Design review of the part built by this model. Coordinates are the model's own, in mm. A direction names the side the tool comes from. Give positions to 0.01 mm unless a question says otherwise; leave off trailing zeros. Loops run counter-clockwise (first coordinate to the right, second up) from the corner with the lowest first, then second, coordinate; pieces in that order, holes last. Notation, with made-up numbers: (-6.75, -25) -> (9.25, -25) arc R33 ccw to (9.25, 7) -> close; hole circle Ø4 at (39, 38). An arc over 180 degrees is marked (long way). Use a Markdown table: item, result. Add a question column.
1. Add section B-B (y = 4.5). State the section outline as (x, z) points, and give its area (3 significant figures).
2. Add section A-A (x = 24). State the section outline as (y, z) points, and give its area (3 significant figures).
3. Add section D-D (x = 13). State the section outline as (y, z) points.
4. For faces 1 (the cylindrical face through (18.797, 6.859, 2.535)), 2 (the flat face through (20, 12.5, 2)), 3 (the flat face through (8, 28, 3)), list the 3-axis set-ups (+Z, -Z, +X, -X, +Y, -Y) from which the entire face can be reached by the end or side of a thin tool; tool diameter is ignored.
5. Add section C-C (z = 4.55). Count the separate pieces of the cut face and the enclosed holes in it, and give its area (3 significant figures).
6. For pin 1 Ø2 at (x, z) = (12.5, 1.5) entering from +Y; pin 2 Ø1.5 at (x, z) = (32, 3.5) entering from -Y; pin 3 Ø1.2 at (y, z) = (1.5, 3.5) entering from +X, all flat-tipped, find the tip position at first contact; note any pin that passes through.
7. Draft analysis for pull direction Y (two halves, no side actions). For faces 4 (the cylindrical face through (10.59, 16.94, 2.46)), 5 (the flat face through (18, 12, 0)), 6 (the flat face through (23.9, 0, 0.8)), state which applies: pulls with the +Y half, pulls with the -Y half, needs draft (parallel to the pull), parting line crosses it, or undercut.
8. To check wall thickness, follow line 1 (X direction, y = 10, z = 2.5); line 2 (Y direction, x = 26.5, z = 3.85); line 3 (X direction, y = 19.5, z = 1.85). State the ranges of each line that lie inside material, in increasing order.
```python
from build123d import *

# Parameters (mm, degrees)
SKETCH1_R           = 2
BOSS_EXTRUDE1_DEPTH = 5
SKETCH2_R           = 1.5
CUT_EXTRUDE1_DEPTH  = 31
CUT_EXTRUDE2_DEPTH  = 6.0000001


with BuildPart() as part:
    # Sketch1 → Boss-Extrude1 (new body)
    with BuildSketch(Plane.XY):
        with BuildLine():
            Line((1, 0), (35, 0))
            ThreePointArc((35, 0), (35.707106781, 0.292893219), (36, 1))
            Line((36, 1), (36, 29))
            ThreePointArc((36, 29), (35.707106781, 29.707106781), (35, 30))
            Line((35, 30), (1, 30))
            ThreePointArc((1, 30), (0.292893219, 29.707106781), (0, 29))
            Line((0, 29), (0, 7))
            Line((0, 7), (0, 1))
            ThreePointArc((0, 1), (0.292893219, 0.292893219), (1, 0))
        make_face()
        with Locations((5, 15)):
            Circle(SKETCH1_R, mode=Mode.SUBTRACT)
        with BuildLine():
            Line((11.967452223, 12.5), (28.032547777, 12.5))
            ThreePointArc((28.032547777, 12.5), (29.423746586, 13.076253414), (30, 14.467452223))
            Line((30, 14.467452223), (30, 15.532547777))
            ThreePointArc((30, 15.532547777), (29.423746586, 16.923746586), (28.032547777, 17.5))
            Line((28.032547777, 17.5), (11.967452223, 17.5))
            ThreePointArc((11.967452223, 17.5), (10.576253414, 16.923746586), (10, 15.532547777))
            Line((10, 15.532547777), (10, 14.467452223))
            ThreePointArc((10, 14.467452223), (10.576253414, 13.076253414), (11.967452223, 12.5))
        make_face(mode=Mode.SUBTRACT)
    extrude(amount=BOSS_EXTRUDE1_DEPTH)

    # Sketch2 → Cut-Extrude1 (cut, through all)
    with BuildSketch(Plane(origin=(0, 30, 0), x_dir=(1, 0, 0), z_dir=(0, 1, 0))):
        with Locations((4, -2.5)):
            Circle(SKETCH2_R)
        with Locations((24, -2.5)):
            Circle(SKETCH2_R)
    extrude(amount=-CUT_EXTRUDE1_DEPTH, mode=Mode.SUBTRACT)

    # Sketch3 → Cut-Extrude2 (cut, through all)
    with BuildSketch(Plane.XY.offset(5)):
        with BuildLine():
            Line((28, 30), (28, 25))
            ThreePointArc((28, 25), (28.292893219, 24.292893219), (29, 24))
            Line((29, 24), (43, 24))
            ThreePointArc((43, 24), (43.707106781, 23.707106781), (44, 23))
            Line((44, 23), (44, 7))
            ThreePointArc((44, 7), (43.707106781, 6.292893219), (43, 6))
            Line((43, 6), (29, 6))
            ThreePointArc((29, 6), (28.292893219, 5.707106781), (28, 5))
            Line((28, 5), (28, 0))
            Line((28, 0), (56.755309453, 0))
            Line((56.755309453, 0), (56.755309453, 30))
            Line((56.755309453, 30), (28, 30))
        make_face()
        with BuildLine():
            Line((8, 30), (8, 26))
            ThreePointArc((8, 26), (9.171572875, 23.171572875), (12, 22))
            Line((12, 22), (16, 22))
            ThreePointArc((16, 22), (18.828427125, 23.171572875), (20, 26))
            Line((20, 26), (20, 30))
            Line((20, 30), (8, 30))
        make_face()
        with BuildLine():
            Line((8, 0), (8, 4))
            ThreePointArc((8, 4), (9.171572875, 6.828427125), (12, 8))
            Line((12, 8), (16, 8))
            ThreePointArc((16, 8), (18.828427125, 6.828427125), (20, 4))
            Line((20, 4), (20, 0))
            Line((20, 0), (8, 0))
        make_face()
    extrude(amount=-CUT_EXTRUDE2_DEPTH, mode=Mode.SUBTRACT)


solid = part.part
```
Taken from the geometry:
| question | item | result |
|---|---|---|
| 1 | outline | (0, 0) -> (8.03, 0) -> (8.03, 5) -> (0, 5) -> close; (19.97, 0) -> (28, 0) -> (28, 5) -> (19.97, 5) -> close; hole circle Ø3 at (4, 2.5); hole circle Ø3 at (24, 2.5) |
| 1 | area | 66.2 mm^2 |
| 2 | outline | (0, 0) -> (12.5, 0) -> (12.5, 1) -> (0, 1) -> close; (0, 4) -> (12.5, 4) -> (12.5, 5) -> (0, 5) -> close; (17.5, 0) -> (30, 0) -> (30, 1) -> (17.5, 1) -> close; (17.5, 4) -> (30, 4) -> (30, 5) -> (17.5, 5) -> close |
| 2 | area | 50.0 mm^2 |
| 3 | outline | (8, 0) -> (12.5, 0) -> (12.5, 5) -> (8, 5) -> close; (17.5, 0) -> (22, 0) -> (22, 5) -> (17.5, 5) -> close |
| 4 | face 1 | +Z, -Z, -Y |
| 4 | face 2 | +Z, -Z |
| 4 | face 3 | +Z, -Z, +Y |
| 5 | separate pieces | 1 |
| 5 | enclosed holes | 2 |
| 5 | area | 696 mm^2 |
| 6 | pin 1 | stops at y = 22.03 |
| 6 | pin 2 | stops at y = 6 |
| 6 | pin 3 | stops at x = 28 |
| 7 | face 4 | undercut |
| 7 | face 5 | needs draft |
| 7 | face 6 | pulls with the -Y half |
| 8 | line 1 | x = 0 to 2.5, 5.5 to 22.5, 25.5 to 36 |
| 8 | line 2 | y = 0 to 12.5, 17.5 to 30 |
| 8 | line 3 | x = 0 to 2.65, 5.35 to 22.65, 25.35 to 36 |
